Build history of the part. All positions in model axes, mm. Round coordinates to 2 decimals unless told otherwise and drop trailing zeros. Write each loop counter-clockwise with the first axis right and the second up, starting at its lowest first coordinate (ties: lowest second). Pieces come first, ordered by that corner, then holes. Notation, with made-up numbers: (43, -24) -> (97, -24) arc R21 ccw to (97, -17) -> close; hole circle Ø3 at (-9.75, -30). An arc over 180 degrees is marked (long way). Answer in a Markdown table with one row per item.
Autodesk Inventor part; units mm, degrees
ref_plane "YZ Plane" through (0, 0, 0) normal (1, 0, 0) x (0, 1, 0)
ref_plane "XZ Plane" through (0, 0, 0) normal (0, 1, 0) x (-1, 0, 0)
ref_plane "XY Plane" through (0, 0, 0) normal (0, 0, 1) x (1, 0, 0)
sketch "Sketch1" plane through (0, 0, 0) normal (0, 0, 1) x (1, 0, 0)
  circle A0 centre (0, 0) radius 11
  circle A1 centre (0, 0) radius 20.6625
  point P0 (16, 0)
  point P1 (0, 16)
  point P2 (-16, 0)
  point P3 (0, -16)
  dimension "d0" = 22
  dimension "d2" = 16
  dimension "d5" = 360
  dimension "d7" = 41.325
extrude "Plate1" add sketch "Sketch1" along normal blind 2 contours A0 | A1
hole "Hole1" at (16, 0, 0) at (0, 16, 0) at (-16, 0, 0) at (0, -16, 0) direction (0, 0, 1) diameter 3.2 end through all
sketch "Sketch2" plane through (0, 0, 0) normal (0, 0, -1) x (-1, 0, 0)
  circle A0 centre (0, 0) radius 5.5
  dimension "d16" = 11
extrude "Cut1" cut sketch "Sketch2" against normal blind 2
equation "\"d14\" = Thickness"
equation "\"d17\" = Thickness"
equation "\"d8\" = Thickness"
equation "\"BendRadius\" = Thickness"
equation "\"BendReliefWidth\" = Thickness"
equation "\"BendReliefDepth\" = 0.5 * Thickness"
equation "\"CornerReliefSize\" = 4 * Thickness"
equation "\"MinimumRemnant\" = 2 * Thickness"
equation "\"TransitionRadius\" = BendRadius"
equation "\"JacobiRadiusSize\" = BendRadius"
equation "\"GapSize\" = Thickness"
properties part number "60mmspacerDicht" material "Aluminum 6061"
Q1. Saw through at C-C on x = -17. Write the cut outline in (y, z).
A:
| item | result |
|---|---|
| outline | (-11.74, 0) -> (-1.25, 0) -> (-1.25, 2) -> (-11.74, 2) -> close; (1.25, 0) -> (11.74, 0) -> (11.74, 2) -> (1.25, 2) -> close |
Q2. Saw through at D-D on y = 15. Write the cut outline in (x, z).
A:
| item | result |
|---|---|
| outline | (-14.21, 0) -> (-1.25, 0) -> (-1.25, 2) -> (-14.21, 2) -> close; (1.25, 0) -> (14.21, 0) -> (14.21, 2) -> (1.25, 2) -> close |
Q3. Saw through at A-A on y = 0. Write the cut outline in (x, z).
A:
| item | result |
|---|---|
| outline | (-20.66, 0) -> (-17.6, 0) -> (-17.6, 2) -> (-20.66, 2) -> close; (-14.4, 0) -> (-5.5, 0) -> (-5.5, 2) -> (-14.4, 2) -> close; (5.5, 0) -> (14.4, 0) -> (14.4, 2) -> (5.5, 2) -> close; (17.6, 0) -> (20.66, 0) -> (20.66, 2) -> (17.6, 2) -> close |
Q4. Drop flat-ended pins along their axis: P1, Ø1, axis at y = -10, z = 1, coming from the -X side; P2, Ø1, axis at y = 13, z = 0.5, coming from the +X side. Give the stop position or say it passes through.
A:
| item | result |
|---|---|
| P1 | x = -18.35 |
| P2 | x = 16.45 |
Q5. Two-plate mould, pull along Y, no slides. Class faces 1 (the cylindrical face through (-4.48, 20.17, 0.99)), 2 (the flat face through (4, -4, 0)), 3 (the cylindrical face through (1.19, -5.37, 0.99)): released by +Y, released by -Y, zero draft, split by the parting line, or undercut.
A:
| item | result |
|---|---|
| face 1 | split by the parting line |
| face 2 | zero draft |
| face 3 | undercut |
Q6. Wall check: line 1 (Y direction, x = 0, z = 0.9); line 2 (Y direction, x = 1, z = 0.1). Give the ranges that are in metal, low to high. Write a range as [from, to].
A:
| item | result |
|---|---|
| line 1 | [-20.66, -17.6], [-14.4, -5.5], [5.5, 14.4], [17.6, 20.66] |
| line 2 | [-20.64, -17.25], [-14.75, -5.41], [5.41, 14.75], [17.25, 20.64] |
